```python
from build123d import *

# Parameters (mm, degrees)
F1_DEPTH = 12.7


with BuildPart() as f1:
    # F0 (on Front) → F1 (new body)
    with BuildSketch(Plane.XZ):
        with BuildLine():
            Line((-25.4, 0), (0, 25.4))
            Line((0, 25.4), (0, 540.721549))
            Line((0, 540.721549), (-25.4, 566.121549))
            Line((-25.4, 566.121549), (-736.6, 566.121549))
            Line((-736.6, 566.121549), (-762, 540.721549))
            ThreePointArc((-762, 540.721549), (-799.197439, 450.918987), (-889, 413.721549))
            Line((-889, 413.721549), (-1447.8, 413.721549))
            Line((-1447.8, 413.721549), (-1473.2, 388.321549))
            Line((-1473.2, 388.321549), (-1473.2, 177.8))
            Line((-1473.2, 177.8), (-1447.8, 152.4))
            Line((-1447.8, 152.4), (-889, 152.4))
            ThreePointArc((-889, 152.4), (-799.197439, 115.202561), (-762, 25.4))
            Line((-762, 25.4), (-736.6, 0))
            Line((-736.6, 0), (-25.4, 0))
        make_face()
    extrude(amount=F1_DEPTH)


solid = f1.part
```
Work out the finished part from the listing and answer in its coordinate system (mm). Round coordinates to 2 decimals unless told otherwise and drop trailing zeros. Write each loop counter-clockwise with the first axis right and the second up, starting at its lowest first coordinate (ties: lowest second). Pieces come first, ordered by that corner, then holes.
1) A cutting plane is placed at C-C on z = 495. Determine the outline of the cut face in (x, y).
2) A cutting plane is placed at B-B on x = -1289. Determine the outline of the cut face in (y, z).
3) Consider probe 1 along Z at (x, y) = (-1361, -7.75); probe 2 along X at (y, z) = (-10, 61.5); probe 3 along X at (y, z) = (-4, 514.5). Determine where each line is inside the solid, lowest interval first.
4) A cutting plane is placed at A-A on y = -2. Determine the outline of the cut face in (x, z).
5) Flat-ended cylindrical pins translate along their axes: P1, Ø1.5, axis at x = -175.5, y = -6.5, coming from the -Z side; P2, Ø6.5, axis at x = -1204, y = -8.5, coming from the +Z side. Find the tip coordinate at first contact, or state that the pin passes through.
Entries:
1. outline: (-770.52, -12.7) - (0, -12.7) - (0, 0) - (-770.52, 0) - close
2. outline: (-12.7, 152.4) - (0, 152.4) - (0, 413.72) - (-12.7, 413.72) - close
3. probe 1: z = 152.4 to 413.72
3. probe 2: x = -767.24 to 0
3. probe 3: x = -764.74 to 0
4. outline: (-1473.2, 177.8) - (-1447.8, 152.4) - (-889, 152.4) arc R127 cw to (-762, 25.4) - (-736.6, 0) - (-25.4, 0) - (0, 25.4) - (0, 540.72) - (-25.4, 566.12) - (-736.6, 566.12) - (-762, 540.72) arc R127 cw to (-889, 413.72) - (-1447.8, 413.72) - (-1473.2, 388.32) - close
5. P1: stops at z = 0
5. P2: stops at z = 413.72
